from build123d import *

# Parameters (mm, degrees)
F2_R     = 7.366
F3_DEPTH = 9.525
F4_R     = 9.525
F5_DEPTH = 1.5875
F8_D     = 9.8044


# Not quite as in the source:
# - a feature of the source that left no trace in its solid (it failed there, or was rolled back) is left out


with BuildPart() as f3:
    # F2 (on Top) → F3 (new body, through all)
    with BuildSketch(Plane.XY):
        Circle(F2_R)
    extrude(amount=-F3_DEPTH)

    # F4 (on Top) → F5 (join, through all)
    with BuildSketch(Plane.XY):
        Circle(F4_R)
    extrude(amount=F5_DEPTH)

    # F8 (through all)
    with Locations(Plane(origin=(0, 0, -9.525), x_dir=(1, 0, 0), z_dir=(0, 0, -1))):
        with Locations((0, 0)):
            Hole(F8_D / 2)


solid = f3.part
Can you work these out from the model? Positions are in its coordinate system, mm. A direction names the side the tool comes from. Round coordinates to 2 decimals unless told otherwise and drop trailing zeros. Loops run counter-clockwise (first coordinate to the right, second up) from the corner with the lowest first, then second, coordinate; pieces in that order, holes last. Notation, with made-up numbers: (-25.75, -35.5) - (-4.75, -35.5) arc R15 cw to (-4.75, -25.5) - close; hole circle Ø11 at (36, 34). An arc over 180 degrees is marked (long way). Use CSV: the item, a comma, the result in double quotes. Start each with the question number.
1) If we section it at C-C on z = -5.25: Write out the boundary of the cut face in (x, y), plus the area to 3 significant figures.
2) We'd pull the mould along Y, two halves only. Please class faces 1 (the cylindrical face through (-4.676, -1.472, -3.891)), 2 (the cylindrical face through (-7.559, -5.796, 0.783)), 3 (the flat face through (5, -2, -9.525)): released by +Y, released by -Y, zero draft, split by the parting line, or undercut.
3) If we section it at D-D on x = 6.75: Write out the boundary of the cut face in (y, z) (1 decimal).
4) If we section it at A-A on x = 0: Write out the boundary of the cut face in (y, z) (1 decimal).
5) For pin 1 Ø1.5 at (x, z) = (5, -6.5) entering from +Y; pin 2 Ø2 at (x, z) = (-2.5, -1.5) entering from +Y; pin 3 Ø3 at (x, z) = (-1, -6) entering from +Y, each with a flat end and sliding along its axis, tell me the tip position at first contact or that it passes through.
6) Please list where these lines run through material, in increasing order: probe 1 along Y at (x, z) = (0, -6); probe 2 along Z at (x, y) = (3.25, -7.75); probe 3 along X at (y, z) = (4.5, -3). Write a range as [from, to].
7) For faces 4 (the cylindrical face through (3.399, -6.535, -4.696)), 5 (the flat face through (4, -4, 1.588)), which set-ups out of +Z, -Z, +X, -X, +Y, -Y let a thin tool reach every point of the face, with its end or its side?
Geometry results:
1,outline,"circle Ø14.73 at (0, 0); hole circle Ø9.8 at (0, 0)"
1,area,"95.0 mm2"
2,face 1,"undercut"
2,face 2,"split by the parting line"
2,face 3,"zero draft"
3,outline,"(-6.7, 0) - (-2.9, 0) - (-2.9, -9.5) - (2.9, -9.5) - (2.9, 0) - (6.7, 0) - (6.7, 1.6) - (-6.7, 1.6) - close"
4,outline,"(-9.5, 0) - (-7.4, 0) - (-7.4, -9.5) - (-4.9, -9.5) - (-4.9, 1.6) - (-9.5, 1.6) - close; (4.9, -9.5) - (7.4, -9.5) - (7.4, 0) - (9.5, 0) - (9.5, 1.6) - (4.9, 1.6) - close"
5,pin 1,"stops at y = 6.02"
5,pin 2,"stops at y = 7.21"
5,pin 3,"stops at y = 7.37"
6,probe 1,"y = [-7.37, -4.9], [4.9, 7.37]"
6,probe 2,"z = [0, 1.59]"
6,probe 3,"x = [-5.83, -1.94], [1.94, 5.83]"
7,face 4,"-Z"
7,face 5,"+Z, +X, -X, +Y, -Y"
